Solid Edge part; units mm, degrees
sketch "Sketch1" plane through (0, 0, 0) normal (0, -1, 0) x (1, 0, 0)
  line L0 (3.5, 2.0207) -> (0, 4.0415)
  line L1 (0, 4.0415) -> (-3.5, 2.0207)
  line L2 (-3.5, 2.0207) -> (-3.5, -2.0207)
  line L3 (-3.5, -2.0207) -> (0, -4.0415)
  line L4 (0, -4.0415) -> (3.5, -2.0207)
  line L5 (3.5, -2.0207) -> (3.5, 2.0207)
extrude "Protrusion1" add sketch "Sketch1" along normal mid plane 3.2
sketch "Sketch2" plane through (0, 0, 0) normal (1, 0, 0) x (0, 1, 0)
  line L0 (-1.6, 2.95) -> (-1.3075, 4.0415)
revolve "RevolvedCutout1" cut sketch "Sketch2" angle 360 about axis through (0, 0, 0) along (0, -1, 0) material side at (0, -1.502, 3.5087)
mirror "Mirror1" about plane through (0, 0, 0) normal (0, -1, 0) of "RevolvedCutout1"
hole "孔_7" at (0, -1.6, 0) direction (0, 1, 0) diameter 3.242 end up to next start chamfer 0.4 start chamfer angle 60 end chamfer 0.4 end chamfer angle 60
Read the model definition and answer for the solid it produces. Units are mm, in the model's axes. Give positions to 0.01 mm unless a question says otherwise; leave off trailing zeros. Write each loop counter-clockwise with the first axis right and the second up, starting at its lowest first coordinate (ties: lowest second). Pieces come first, ordered by that corner, then holes. Notation, with made-up numbers: (26, -13.75) -> (50, -13.75) arc R23 cw to (50, 0.25) -> close; hole circle Ø9 at (-33, -39). An arc over 180 degrees is marked (long way). Answer as a JSON object with one key per item and string values.
1) For a pull along Z with two mould halves and no side action, classify faces 1 (the cylindrical face through (-1.438, -0.019, -0.748)), 2 (the flat face through (-1.726, 0.02, 3.045)), 3 (the flat face through (3.5, 0, 0)), 4 (the flat face through (1.726, 0.02, -3.045)) as pulls with the +Z half, pulls with the -Z half, needs draft (parallel to the pull), parting line crosses it, or undercut.
Findings below:
{"face 1": "undercut", "face 2": "pulls with the +Z half", "face 3": "needs draft", "face 4": "pulls with the -Z half"}
2) Straight lines are drawn through the part: probe 1 along X at (y, z) = (0.7, 0); probe 2 along Y at (x, z) = (1, -1.75); probe 3 along X at (y, z) = (0.9, -0.5). For each, find the intervals that lie inside material, in ascending order. Write a range as from..to.
Findings below:
{"probe 1": "x = -3.5..-1.62, 1.62..3.5", "probe 2": "y = -1.6..1.6", "probe 3": "x = -3.5..-1.54, 1.54..3.5"}
3) Flat-ended cylindrical pins translate along their axes: pin 1 Ø4 at (x, z) = (0, 0) entering from +Y; pin 2 Ø2 at (x, z) = (0, 1) entering from -Y; pin 3 Ø1.5 at (x, y) = (2, -0.5) entering from +Z. Find the tip coordinate at first contact, or state that the pin passes through.
Findings below:
{"pin 1": "stops at y = 1.59", "pin 2": "stops at y = -1.59", "pin 3": "stops at z = 3.32"}
4) Section B-B on y = 0.2 is taken. Write down the section's boundary in (x, z), then the cut area to 3 significant figures.
Findings below:
{"outline": "(-3.5, -2.02) -> (0, -4.04) -> (3.5, -2.02) -> (3.5, 2.02) -> (0, 4.04) -> (-3.5, 2.02) -> close; hole circle Ø3.24 at (0, 0)", "area": "34.2 mm^2"}
5) Section A-A on z = 0 is taken. Write down the section's boundary in (x, y), then the cut area to 3 significant figures.
Findings below:
{"outline": "(-3.5, -1.45) -> (-2.95, -1.6) -> (-2.02, -1.6) -> (-1.62, -1.37) -> (-1.62, 1.37) -> (-2.02, 1.6) -> (-2.95, 1.6) -> (-3.5, 1.45) -> close; (1.62, -1.37) -> (2.02, -1.6) -> (2.95, -1.6) -> (3.5, -1.45) -> (3.5, 1.45) -> (2.95, 1.6) -> (2.02, 1.6) -> (1.62, 1.37) -> close", "area": "11.7 mm^2"}
